Build history of the part. All positions in model axes, mm. Face numbers are marked on the shaded views. A direction names the side the tool comes from. Round coordinates to 2 decimals unless told otherwise and drop trailing zeros. Write each loop counter-clockwise with the first axis right and the second up, starting at its lowest first coordinate (ties: lowest second). Pieces come first, ordered by that corner, then holes. Notation, with made-up numbers: (76.5, 3.5) -> (132.5, 3.5) arc R32 cw to (132.5, 42.5) -> close; hole circle Ø6 at (-22, 59). An arc over 180 degrees is marked (long way). Answer in a Markdown table with one row per item.
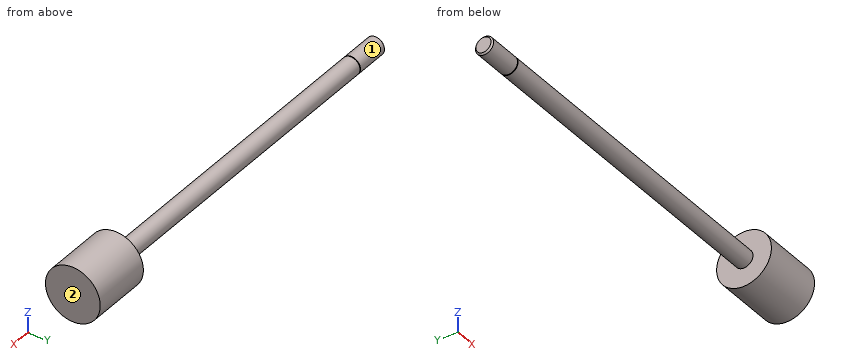
```python
from build123d import *

# Parameters (mm, degrees)
SKETCH3_W = 0.254
SKETCH3_H = 0.508


with BuildPart() as part:
    # Sketch1 → Revolve1 (revolve)
    with BuildSketch(Plane.XY):
        Polygon((0, 0), (0, 3.175), (116.6876, 3.175), (116.6876, 9.62025), (138.1252, 9.62025), (138.1252, 0), align=None)
    revolve(axis=Axis((138.1252, 0, 0), (-1, 0, 0)))

    # Sketch2 → Revolve2 (revolve)
    with BuildSketch(Plane.XY):
        Polygon((-12.7, 0), (-12.7, 2.63398), (-12.15898, 3.175), (0, 3.175), (0, 0), align=None)
    revolve(axis=Axis((0, 0, 0), (-1, 0, 0)))

    # Sketch3 → Cut-Revolve1 (revolve, cut)
    with BuildSketch(Plane.XY):
        with Locations((-0.127, 3.175)):
            Rectangle(SKETCH3_W, SKETCH3_H)
    revolve(axis=Axis((0, 0, 0), (-1, 0, 0)), mode=Mode.SUBTRACT)


solid = part.part
```
Q1. Saw through at A-A on y = 0. Write the cut outline in (x, z) (3 decimals).
A:
| item | result |
|---|---|
| outline | (-12.7, -2.634) -> (-12.159, -3.175) -> (-0.254, -3.175) -> (-0.254, -2.921) -> (0, -2.921) -> (0, -3.175) -> (116.688, -3.175) -> (116.688, -9.62) -> (138.125, -9.62) -> (138.125, 9.62) -> (116.688, 9.62) -> (116.688, 3.175) -> (0, 3.175) -> (0, 2.921) -> (-0.254, 2.921) -> (-0.254, 3.175) -> (-12.159, 3.175) -> (-12.7, 2.634) -> close |
Q2. Wall check: line 1 (X direction, y = -6.25, z = -1); line 2 (Z direction, x = 17, y = 1.75); line 3 (Y direction, x = 113.5, z = 0.75). Give the ranges that are in metal, low to high. Write a range as [from, to].
A:
| item | result |
|---|---|
| line 1 | [116.69, 138.13] |
| line 2 | [-2.65, 2.65] |
| line 3 | [-3.09, 3.09] |
Q3. Saw through at C-C on x = 46.5. Write the cut outline in (y, z) (3 decimals), plus the area to 3 significant figures.
A:
| item | result |
|---|---|
| outline | circle Ø6.35 at (0, 0) |
| area | 31.7 mm² |
Q4. Saw through at D-D on y = 7.5. Write the cut outline in (x, z), plus the area to 3 significant figures.
A:
| item | result |
|---|---|
| outline | (116.69, -6.02) -> (138.13, -6.02) -> (138.13, 6.02) -> (116.69, 6.02) -> close |
| area | 258 mm² |
Q5. Drop flat-ended pins along their axis: P1, Ø8, axis at x = 11.5, y = -7.5, coming from the +Z side; P2, Ø10, axis at x = 103.5, y = 6, coming from the -Z side; P3, Ø5, axis at x = 56, y = -4, coming from the +Z side; P4, Ø10, axis at x = 64.5, z = -4.5, coming from the -Y side (3 decimals). Give the stop position or say it passes through.
A:
| item | result |
|---|---|
| P1 | through |
| P2 | z = -3.01 |
| P3 | z = 2.8 |
| P4 | y = -3.175 |
Q6. Which spindle directions (+Z, -Z, +X, -X, +Y, -Y) get a long thin tool onto all of the face, cutting with end or side? Do the marked faces 1 and 2. Say none if no direction does.
A:
| item | result |
|---|---|
| face 1 | -X |
| face 2 | +Z, -Z, +X, +Y, -Y |
